CAD build for the part. Positions are in the model's coordinates, mm. A direction names the side the tool comes from. Coordinates: 2 decimals unless noted, no trailing zeros. Write each loop counter-clockwise with the first axis right and the second up, starting at its lowest first coordinate (ties: lowest second). Pieces come first, ordered by that corner, then holes.
```python
from build123d import *

# Parameters (mm, degrees)
BOSS_EXTRUDE1_DEPTH     = 10
CUT_EXTRUDE1_DEPTH      = 23.974660823
CUT_EXTRUDE1_DEPTH_BACK = 23.974660823
SKETCH2_R               = 1.5


with BuildPart() as part:
    # Sketch1 → Boss-Extrude1 (new body)
    with BuildSketch(Plane.XY):
        Polygon((-16.088351064, -3.521010638), (-16.088351064, -1.521010638), (-10.088351064, -1.521010638), (-10.088351064, 11.478989362), (8.331648936, 11.478989362), (8.331648936, -1.521010638), (14.331648936, -1.521010638), (14.331648936, -3.521010638), (6.331648936, -3.521010638), (6.331648936, 9.478989362), (-8.088351064, 9.478989362), (-8.088351064, -3.521010638), align=None)
    extrude(amount=BOSS_EXTRUDE1_DEPTH)

    # Sketch2 → Cut-Extrude1 (cut, two sides: drawn at the far end of the back side and taken through both)
    with BuildSketch(Plane(origin=(0, -1.521010638, 0), x_dir=(1, 0, 0), z_dir=(0, 1, 0)).offset(-CUT_EXTRUDE1_DEPTH_BACK)):
        with Locations(Location((-13.088351064, -5, 0), (0, 0, 270))):
            Circle(SKETCH2_R)
        with Locations(Location((11.112056512, -5, 0), (0, 0, 270))):
            Circle(SKETCH2_R)
    extrude(amount=CUT_EXTRUDE1_DEPTH + CUT_EXTRUDE1_DEPTH_BACK, mode=Mode.SUBTRACT)


solid = part.part
```
Item 1: Flat gauge pins, fed straight in: pin 1 Ø1 at (y, z) = (1, 8) entering from +X; pin 2 Ø5 at (y, z) = (3, 3.5) entering from -X; pin 3 Ø1.8 at (x, z) = (-14, 4.5) entering from +Y. Where does each tip first touch, or does it go through?
Item 2: Saw through at A-A, the plane y = 3.75. Write the cut outline in (x, z).
Item 3: Wall check: line 1 along X through (y, z) = (-2.95, 5); line 2 along X through (y, z) = (-1, 1.25); line 3 along X through (y, z) = (-2.5, 8). Give the ranges that are in metal, low to high.
Item 4: Saw through at B-B, the plane z = 5. Write the cut outline in (x, y), and give its area (3 significant figures).
Item 5: Two-plate mould, pull along Z, no slides. Class faces 1 (the cylindrical face through (-11.824, -2.535, 5.806)), 2 (the flat face through (-1, 10, 10)), 3 (the flat face through (-10.088, 5, 5)): +Z half, -Z half, draft (parallel to the pull), parting line (faces both ways), or undercut.
Item 6: Saw through at D-D, the plane z = 1.25. Write the cut outline in (x, y).
Item 7: Saw through at C-C, the plane x = -12.5. Write the cut outline in (y, z).
Item 8: Which spindle directions (+Z, -Z, +X, -X, +Y, -Y) get a long thin tool onto all of the face, cutting with end or side? Do faces 4 (the flat face through (14.332, -3, 5)), 5 (the flat face through (-11, -3.521, 5)), 6 (the flat face through (-1, 9.479, 5)), 7 (the flat face through (-11.8, -1.521, 3.8)), 8 (the flat face through (8.332, 5, 5)). Say none if no direction does.
Working result:
1. pin 1: stops at x = 8.33
1. pin 2: stops at x = -10.09
1. pin 3: stops at y = -1.52
2. outline: (-10.09, 0) - (-8.09, 0) - (-8.09, 10) - (-10.09, 10) - close; (6.33, 0) - (8.33, 0) - (8.33, 10) - (6.33, 10) - close
3. line 1: x = -16.09 to -14.59, -11.59 to -8.09, 6.33 to 9.61, 12.61 to 14.33
3. line 2: x = -10.09 to -8.09, 6.33 to 8.33
3. line 3: x = -16.09 to -8.09, 6.33 to 14.33
4. outline: (-16.09, -3.52) - (-14.59, -3.52) - (-14.59, -1.52) - (-16.09, -1.52) - close; (-11.59, -3.52) - (-8.09, -3.52) - (-8.09, 9.48) - (6.33, 9.48) - (6.33, -3.52) - (9.61, -3.52) - (9.61, -1.52) - (8.33, -1.52) - (8.33, 11.48) - (-10.09, 11.48) - (-10.09, -1.52) - (-11.59, -1.52) - close; (12.61, -3.52) - (14.33, -3.52) - (14.33, -1.52) - (12.61, -1.52) - close
4. area: 101 mm2
5. face 1: undercut
5. face 2: +Z half
5. face 3: draft
6. outline: (-16.09, -3.52) - (-8.09, -3.52) - (-8.09, 9.48) - (6.33, 9.48) - (6.33, -3.52) - (14.33, -3.52) - (14.33, -1.52) - (8.33, -1.52) - (8.33, 11.48) - (-10.09, 11.48) - (-10.09, -1.52) - (-16.09, -1.52) - close
7. outline: (-3.52, 0) - (-1.52, 0) - (-1.52, 3.62) - (-3.52, 3.62) - close; (-3.52, 6.38) - (-1.52, 6.38) - (-1.52, 10) - (-3.52, 10) - close
8. face 4: +Z, -Z, +X, +Y, -Y
8. face 5: +Z, -Z, +X, -X, -Y
8. face 6: +Z, -Z, -Y
8. face 7: +Z, -Z, -X, +Y
8. face 8: +Z, -Z, +X, +Y
